from build123d import *

# Parameters (mm, degrees)
F0_W       = 2000
F0_H       = 750
F1_DEPTH   = 200
F2_T       = -18
F3_W       = 18
F3_H       = 714
F4_DEPTH   = 182
F6_DEPTH   = 25
F7_W       = 150
F7_H       = 88.6
F7_W_2     = 160
F7_H_2     = 45
F8_DEPTH   = 25
F9_DEPTH   = 25
F10_DEPTH  = 25
F11_W      = 360
F11_H      = 120
F12_DEPTH  = 25
F12_FACE_W = 360
F12_FACE_H = 120
F13_DEPTH  = 25
F14_DEPTH  = 25
F15_W      = 360
F15_H      = 120
F16_DEPTH  = 20


with BuildPart() as f1:
    # F0 (on Top) → F1 (new body)
    with BuildSketch(Plane.XY):
        Rectangle(F0_W, F0_H)
    extrude(amount=F1_DEPTH)

    # F2
    f2_openings = [f1.faces().sort_by_distance(p)[0] for p in [
        (0, 0, 200),
    ]]
    offset(amount=F2_T, openings=f2_openings)

    # F3 (on face) → F4 (join)
    with BuildSketch(Plane.XY.offset(18)):
        with Locations((-9, 0)):
            Rectangle(F3_W, F3_H)
    extrude(amount=F4_DEPTH)

    # F5 (on face) → F6 (cut)
    with BuildSketch(Plane(origin=(-18, 0, 0), x_dir=(0, -1, 0), z_dir=(-1, 0, 0))):
        Polygon((250, 169), (0, 169), (-250, 169), (-250, 49), (250, 49), align=None)
    extrude(amount=-F6_DEPTH, mode=Mode.SUBTRACT)

    # F7 (on face) → F8 (cut)
    with BuildSketch(Plane(origin=(0, -357, 0), x_dir=(-1, 0, 0), z_dir=(0, 1, 0))):
        with Locations((907, 62.3)):
            Rectangle(F7_W, F7_H)
        Polygon((103.00435, 28), (143.00435, 28), (140.777453, 137.977456), (100.777453, 137.977456), align=None)
        with Locations((248, 50.5)):
            Rectangle(F7_W_2, F7_H_2)
    extrude(amount=-F8_DEPTH, mode=Mode.SUBTRACT)

    # F7 (on face) → F9 (cut)
    with BuildSketch(Plane(origin=(0, -357, 0), x_dir=(-1, 0, 0), z_dir=(0, 1, 0))):
        with Locations((907, 62.3)):
            Rectangle(F7_W, F7_H)
        Polygon((103.00435, 28), (143.00435, 28), (140.777453, 137.977456), (100.777453, 137.977456), align=None)
        with Locations((248, 50.5)):
            Rectangle(F7_W_2, F7_H_2)
    extrude(amount=-F9_DEPTH, mode=Mode.SUBTRACT)

    # F7 (on face) → F10 (cut)
    with BuildSketch(Plane(origin=(0, -357, 0), x_dir=(-1, 0, 0), z_dir=(0, 1, 0))):
        with Locations((907, 62.3)):
            Rectangle(F7_W, F7_H)
        Polygon((103.00435, 28), (143.00435, 28), (140.777453, 137.977456), (100.777453, 137.977456), align=None)
        with Locations((248, 50.5)):
            Rectangle(F7_W_2, F7_H_2)
    extrude(amount=-F10_DEPTH, mode=Mode.SUBTRACT)

    # F11 (on face) → F12 (join)
    with BuildSketch(Plane(origin=(982, 0, 0), x_dir=(0, -1, 0), z_dir=(-1, 0, 0))):
        with Locations((0, 109)):
            Rectangle(F11_W, F11_H)
    extrude(amount=F12_DEPTH)

    # F12_face (on face) → F13 (cut)
    with BuildSketch(Plane(origin=(957, 0, 109), x_dir=(0, -1, 0), z_dir=(-1, 0, 0))):
        Rectangle(F12_FACE_W, F12_FACE_H)
    extrude(amount=-F13_DEPTH, mode=Mode.SUBTRACT)

    # F11 (on face) → F14 (cut)
    with BuildSketch(Plane(origin=(982, 0, 0), x_dir=(0, -1, 0), z_dir=(-1, 0, 0))):
        with Locations((0, 109)):
            Rectangle(F11_W, F11_H)
    extrude(amount=-F14_DEPTH, mode=Mode.SUBTRACT)

    # F15 (on face) → F16 (cut)
    with BuildSketch(Plane(origin=(-1000, 0, 0), x_dir=(0, -1, 0), z_dir=(-1, 0, 0))):
        with Locations((-0.642158, 109.018745)):
            Rectangle(F15_W, F15_H)
    extrude(amount=-F16_DEPTH, mode=Mode.SUBTRACT)


solid = f1.part
Design review of the part built by this model. Coordinates are the model's own, in mm. A direction names the side the tool comes from. Give positions to 0.01 mm unless a question says otherwise; leave off trailing zeros. Order: outer loops, then holes, each group sorted by start corner. A loop starts at its lowest first (then second) coordinate and runs counter-clockwise, first axis right, second up.
1. Add section D-D, the plane x = 335.5. State the section outline as (y, z) points, then the cut area to 3 significant figures.
Solution:
outline: (-375, 0) - (375, 0) - (375, 200) - (357, 200) - (357, 18) - (-357, 18) - (-357, 200) - (-375, 200) - close
area: 20,100 mm2
2. Tool access review of faces 4 (the flat face through (0, -5, 47)), 5 (the flat face through (-14, 5, 0)): name each direction out of +Z, -Z, +X, -X, +Y, -Y from which nothing blocks a thin tool from reaching the whole face with its end or side.
Solution:
face 4: +Z
face 5: -Z, +X, -X, +Y, -Y
3. Mouldability with a two-part tool opening along Y and no side actions: class faces 1 (the flat face through (-1000, -5, 32)), 2 (the flat face through (-14, 375, 99)), 3 (the flat face through (-18, -5, 47)) as +Y half, -Y half, draft (parallel to the pull), parting line (faces both ways), or undercut.
Solution:
face 1: draft
face 2: +Y half
face 3: undercut
4. Add section A-A, the plane y = -219. State the section outline as (x, z) points, then the cut area to 3 significant figures.
Solution:
outline: (-1000, 0) - (1000, 0) - (1000, 200) - (982, 200) - (982, 18) - (0, 18) - (0, 49) - (-18, 49) - (-18, 18) - (-982, 18) - (-982, 200) - (-1000, 200) - close; (-18, 169) - (0, 169) - (0, 200) - (-18, 200) - close
area: 43,700 mm2
5. For pin 1 Ø8 at (x, y) = (191, 103.5) entering from +Z, flat-tipped, find the tip position at first contact; note if it passes through.
Solution:
pin 1: stops at z = 18
6. To check wall thickness, follow L1, parallel to X at y = -259, z = 136.5; L2, parallel to Y at x = -14.5, z = 58.5; L3, parallel to Y at x = -706, z = 57.5. State the ranges of each line that lie inside material, in increasing order.
Solution:
L1: x = -1000 to -982, -18 to 0, 982 to 1000
L2: y = -375 to -250, 250 to 375
L3: y = -375 to -357, 357 to 375
7. Add section B-B, the plane y = 145. State the section outline as (x, z) points, then the cut area to 3 significant figures.
Solution:
outline: (-1000, 0) - (1000, 0) - (1000, 49) - (982, 49) - (982, 18) - (0, 18) - (0, 49) - (-18, 49) - (-18, 18) - (-982, 18) - (-982, 49.02) - (-1000, 49.02) - close; (-1000, 169.02) - (-982, 169.02) - (-982, 200) - (-1000, 200) - close; (-18, 169) - (0, 169) - (0, 200) - (-18, 200) - close; (982, 169) - (1000, 169) - (1000, 200) - (982, 200) - close
area: 39,300 mm2
8. Add section C-C, the plane x = -255.5. State the section outline as (y, z) points, then the cut area to 3 significant figures.
Solution:
outline: (-375, 0) - (375, 0) - (375, 200) - (357, 200) - (357, 18) - (-357, 18) - (-357, 28) - (-375, 28) - close; (-375, 73) - (-357, 73) - (-357, 200) - (-375, 200) - close
area: 19,200 mm2
